Verification items for the finished model (mm, model axes). Face numbers are marked on the shaded views. Round coordinates to 2 decimals unless told otherwise and drop trailing zeros. Order: outer loops, then holes, each group sorted by start corner. A loop starts at its lowest first (then second) coordinate and runs counter-clockwise, first axis right, second up. Notation, with made-up numbers: (-15.5, 75.25) -> (6.5, 75.25) arc R20 ccw to (6.5, 87.25) -> close; hole circle Ø11 at (59.25, -30). An arc over 180 degrees is marked (long way). Return JSON: item names as keys, results as strings. Group by question number.
Item 1: Sectioned sample at D-D on z = 10. Record the cut outline in (x, y), plus the area to 3 significant figures.
Item 2: Scan lines: probe 1 along X at (y, z) = (0.75, 0); probe 2 along X at (y, z) = (-1.75, 0); probe 3 along Z at (x, y) = (17.5, 0.25). Record each from-to range of solid material in increasing order. Write a range as from..to.
Item 3: Sectioned sample at C-C on y = 1.75. Record the cut outline in (x, z).
Item 4: Draft check along Z on the marked faces 1, 2 and 3. Enter one of: pulls with the +Z half, pulls with the -Z half, needs draft (parallel to the pull), parting line crosses it, or undercut.
Item 5: Sectioned sample at A-A on x = 0. Record the cut outline in (y, z).
Item 6: Depth check by flat-ended pin: pin 1 Ø2 at (y, z) = (-3, -19.5) entering from +X; pin 2 Ø10 at (x, z) = (32, -4.5) entering from -Y; pin 3 Ø5 at (y, z) = (-1.5, 12.5) entering from -X; pin 4 Ø6.5 at (x, z) = (-21.25, 36.81) entering from +Y. Enter the tip coordinate at first touch or a pass-through.
Item 7: Sectioned sample at B-B on z = 0. Record the cut outline in (x, y), plus the area to 3 significant figures.
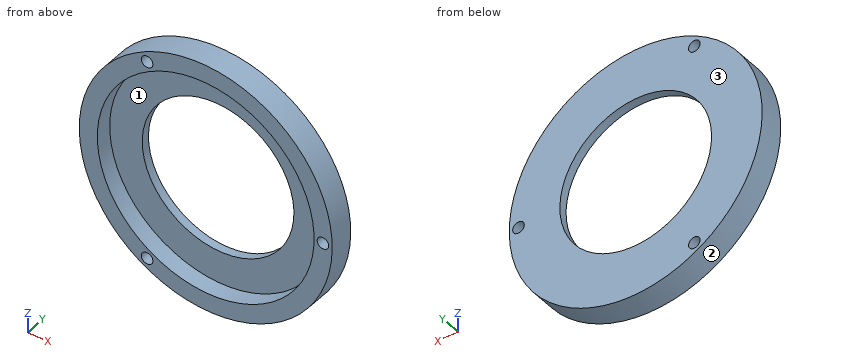
```python
from build123d import *

# Parameters (mm, degrees)
SKETCH1_R           = 45.85
SKETCH1_R_2         = 2.1
SKETCH1_R_3         = 39.3
BOSS_EXTRUDE1_DEPTH = 6
BOSS_EXTRUDE2_START = 3
SKETCH1_4_R         = 45.85
SKETCH1_4_R_2       = 2.1
SKETCH1_4_R_3       = 27.5
BOSS_EXTRUDE2_DEPTH = 3


with BuildPart() as part:
    # Sketch1 → Boss-Extrude1 (new body)
    with BuildSketch(Plane(origin=(0, 0, 0), x_dir=(1, 0, 0), z_dir=(0, 1, 0))):
        with Locations(Location((0, 0, 0), (0, 0, 270))):
            Circle(SKETCH1_R)
        with Locations(Location((42.5, 0, 0), (0, 0, 270))):
            Circle(SKETCH1_R_2, mode=Mode.SUBTRACT)
        with Locations(Location((-21.25, -36.806079661, 0), (0, 0, 270))):
            Circle(SKETCH1_R_2, mode=Mode.SUBTRACT)
        with Locations(Location((-21.25, 36.806079661, 0), (0, 0, 270))):
            Circle(SKETCH1_R_2, mode=Mode.SUBTRACT)
        with Locations(Location((0, 0, 0), (0, 0, 270))):
            Circle(SKETCH1_R_3, mode=Mode.SUBTRACT)
    extrude(amount=-BOSS_EXTRUDE1_DEPTH)

    # Sketch1_4 → Boss-Extrude2 (add)
    with BuildSketch(Plane(origin=(0, 0, 0), x_dir=(1, 0, 0), z_dir=(0, 1, 0)).offset(BOSS_EXTRUDE2_START)):
        with Locations(Location((0, 0, 0), (0, 0, 270))):
            Circle(SKETCH1_4_R)
        with Locations(Location((-21.25, -36.806079661, 0), (0, 0, 270))):
            Circle(SKETCH1_4_R_2, mode=Mode.SUBTRACT)
        with Locations(Location((-21.25, 36.806079661, 0), (0, 0, 270))):
            Circle(SKETCH1_4_R_2, mode=Mode.SUBTRACT)
        with Locations(Location((42.5, 0, 0), (0, 0, 270))):
            Circle(SKETCH1_4_R_2, mode=Mode.SUBTRACT)
        with Locations(Location((0, 0, 0), (0, 0, 270))):
            Circle(SKETCH1_4_R_3, mode=Mode.SUBTRACT)
    extrude(amount=-BOSS_EXTRUDE2_DEPTH)


solid = part.part
```
Recorded:
{
 "1": {"outline": "(-44.75, -6) -> (-38.01, -6) -> (-38.01, 0) -> (-25.62, 0) -> (-25.62, 3) -> (-44.75, 3) -> close; (25.62, 0) -> (38.01, 0) -> (38.01, -6) -> (44.75, -6) -> (44.75, 3) -> (25.62, 3) -> close", "area": "196 mm²"},
 "2": {"probe 1": "-45.85..-27.5, 27.5..40.4, 44.6..45.85", "probe 2": "-45.85..-39.3, 39.3..40.4, 44.6..45.85", "probe 3": "-42.38..-21.21, 21.21..42.38"},
 "3": {"outline": "circle Ø91.7 at (0, 0); hole circle Ø55 at (0, 0); hole circle Ø4.2 at (-21.25, -36.81); hole circle Ø4.2 at (-21.25, 36.81); hole circle Ø4.2 at (42.5, 0)"},
 "4": {"face 1": "undercut", "face 2": "parting line crosses it", "face 3": "needs draft"},
 "5": {"outline": "(-6, -45.85) -> (3, -45.85) -> (3, -27.5) -> (0, -27.5) -> (0, -39.3) -> (-6, -39.3) -> close; (-6, 39.3) -> (0, 39.3) -> (0, 27.5) -> (3, 27.5) -> (3, 45.85) -> (-6, 45.85) -> close"},
 "6": {"pin 1": "x = 41.95", "pin 2": "y = 0", "pin 3": "x = -44.75", "pin 4": "y = 3"},
 "7": {"outline": "(-45.85, -6) -> (-39.3, -6) -> (-39.3, 0) -> (-27.5, 0) -> (-27.5, 3) -> (-45.85, 3) -> close; (27.5, 0) -> (39.3, 0) -> (39.3, -6) -> (40.4, -6) -> (40.4, 3) -> (27.5, 3) -> close; (44.6, -6) -> (45.85, -6) -> (45.85, 3) -> (44.6, 3) -> close", "area": "151 mm²"}
}
